Could you check a few things on this drawing? It's one solid part, dimensions in mm from its lowest x, y, z. A direction names the side the tool comes from. Give positions to 0.01 mm unless a question says otherwise; leave off trailing zeros. Loops run counter-clockwise (first coordinate to the right, second up) from the corner with the lowest first, then second, coordinate; pieces in that order, holes last. Notation, with made-up numbers: M 66.25,16 L 91.25,16 A37 ccw 91.25,52 Z; hole C -31.75,70 d3. An arc over 180 degrees is marked long. Answer as CSV lines item,"result". Start each with the question number.
Item 1: Will these pins go through, and if not, where does the flat tip stop? P1, Ø5, axis at x = 60.5, z = 36.5, coming from the -Y side; P2, Ø22, axis at y = 24, z = 26, coming from the -X side; P3, Ø4, axis at y = 28.5, z = 54, coming from the +X side.
Item 2: If I drill on line 1 along Y through (x, z) = (30, 50); line 2 along X through (y, z) = (24.5, 42.5); line 3 along Y through (x, z) = (75, 31.5), over which ranges is the centre line in solid material (lowest first)? Write a range as from..to.
Item 3: If we mould it in two halves opening along X, with no side actions, what happens to the marked faces 1, 2 and 3? For each: released by +X, released by -X, zero draft, split by the parting line, or undercut.
Item 4: For the marked faces 4, 5 and 6, which set-ups out of +Z, -Z, +X, -X, +Y, -Y let a thin tool reach every point of the face, with its end or its side?
Item 5: I want a section at A-A on x = 48.5. List the corners of the cut face in (y, z) for me.
Item 6: I want a section at D-D on y = 39. List the corners of the cut face in (x, z) for me.
Item 7: I want a section at C-C on z = 24.5. List the corners of the cut face in (x, y) for me.
Item 8: I want a section at B-B on y = 25.5. List the corners of the cut face in (x, z) for me, plus the area to 3 significant figures.
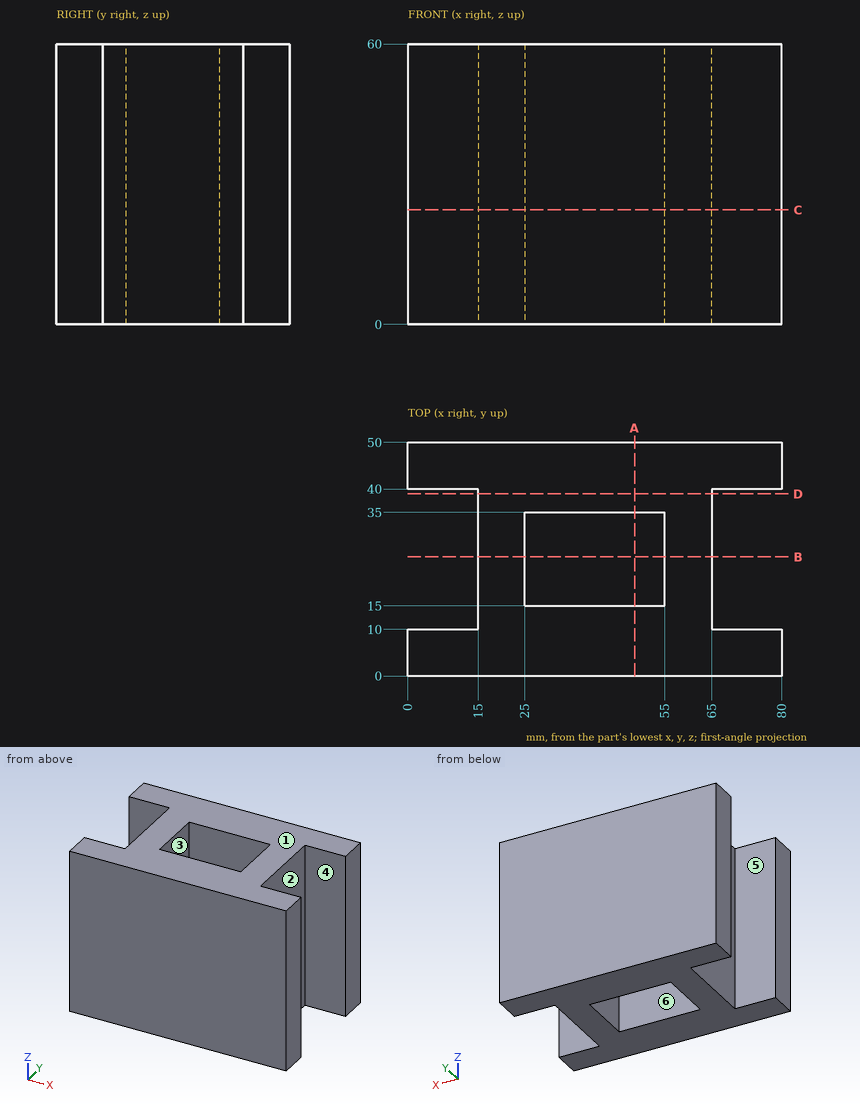
Result:
1,P1,"y = 0"
1,P2,"x = 15"
1,P3,"x = 65"
2,line 1,"0..15, 35..50"
2,line 2,"15..25, 55..65"
2,line 3,"0..10, 40..50"
3,face 1,"zero draft"
3,face 2,"released by +X"
3,face 3,"undercut"
4,face 4,"+Z, -Z, +X"
4,face 5,"+Z, -Z, -X"
4,face 6,"+Z, -Z"
5,outline,"M 0,0 L 15,0 L 15,60 L 0,60 Z; M 35,0 L 50,0 L 50,60 L 35,60 Z"
6,outline,"M 15,0 L 65,0 L 65,60 L 15,60 Z"
7,outline,"M 0,0 L 80,0 L 80,10 L 65,10 L 65,40 L 80,40 L 80,50 L 0,50 L 0,40 L 15,40 L 15,10 L 0,10 Z; hole M 25,15 L 55,15 L 55,35 L 25,35 Z"
8,outline,"M 15,0 L 25,0 L 25,60 L 15,60 Z; M 55,0 L 65,0 L 65,60 L 55,60 Z"
8,area,"1,200 mm^2"
